Here's the drawing with two shaded views (mm, measured from the low corner). I have some questions. A direction names the side the tool comes from. Give positions to 0.01 mm unless a question says otherwise; leave off trailing zeros. Loops run counter-clockwise (first coordinate to the right, second up) from the corner with the lowest first, then second, coordinate; pieces in that order, holes last. Notation, with made-up numbers: M 56,49.5 L 112,49.5 A10 ccw 112,65.5 Z; hole C 40.25,20.25 d8. An arc over 180 degrees is marked long. Use a Markdown table: item, result. Add a question column.
1) Which directions (+Z, -Z, +X, -X, +Y, -Y) give clear straight access to the entire face, cutting with the end or side of a thin tool? Please do the marked faces 4, 5 and 6.
2) If I drill on line 1 along Z through (x, y) = (37.5, 3.5); line 2 along Z through (x, y) = (47.5, 22.5); line 3 along X through (y, z) = (36.5, 5), over which ranges is the centre line in solid material (lowest first)? Write a range as [from, to].
3) We'd pull the mould along Z, two halves only. Please class the marked faces 1, 2 and 3: +Z half, -Z half, draft (parallel to the pull), parting line (faces both ways), or undercut.
4) Suppose I cut it at A-A on x = 34. List the corners of the cut face in (y, z) for me.
5) Will these pins go through, and if not, where does the flat tip stop? pin 1 Ø9.5 at (x, y) = (16.5, 5.5) entering from -Z; pin 2 Ø0.9 at (y, z) = (37, 5.5) entering from +X; pin 3 Ø2 at (x, z) = (61.5, 19) entering from +Y.
6) Suppose I cut it at D-D on z = 19.5. List the corners of the cut face in (x, y) for me.
7) Suppose I cut it at C-C on y = 24.5. List the corners of the cut face in (x, z) for me.
8) Suppose I cut it at B-B on z = 12. List the corners of the cut face in (x, y) for me.
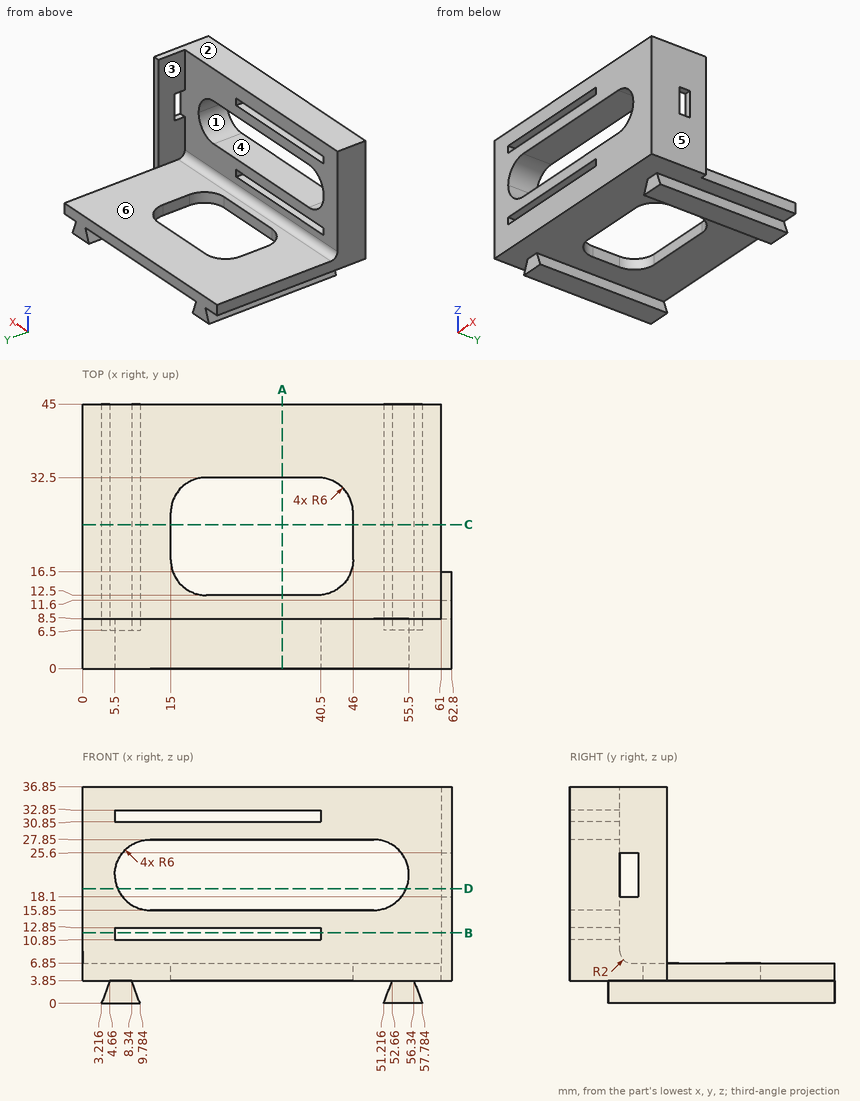
Answer block:
| question | item | result |
|---|---|---|
| 1 | face 4 | +Y, -Y |
| 1 | face 5 | +Z, -Z, +X, +Y, -Y |
| 1 | face 6 | +Z, -X, +Y |
| 2 | line 1 | z = [3.85, 10.85], [12.85, 15.85], [27.85, 30.85], [32.85, 36.85] |
| 2 | line 2 | z = [3.85, 6.85] |
| 2 | line 3 | x = [0, 61] |
| 3 | face 1 | undercut |
| 3 | face 2 | +Z half |
| 3 | face 3 | draft |
| 4 | outline | M 0,3.85 L 12.5,3.85 L 12.5,6.85 L 10.5,6.85 A2 cw 8.5,8.85 L 8.5,10.85 L 0,10.85 Z; M 0,12.85 L 8.5,12.85 L 8.5,15.85 L 0,15.85 Z; M 0,27.85 L 8.5,27.85 L 8.5,30.85 L 0,30.85 Z; M 0,32.85 L 8.5,32.85 L 8.5,36.85 L 0,36.85 Z; M 32.5,3.85 L 45,3.85 L 45,6.85 L 32.5,6.85 Z |
| 5 | pin 1 | stops at z = 3.85 |
| 5 | pin 2 | stops at x = 61 |
| 5 | pin 3 | stops at y = 16.5 |
| 6 | outline | M 0,0 L 5.98,0 L 5.98,8.5 L 0,8.5 Z; M 55.02,0 L 62.8,0 L 62.8,8.5 L 55.02,8.5 Z; M 61,11.6 L 62.8,11.6 L 62.8,16.5 L 61,16.5 Z |
| 7 | outline | M 0,3.85 L 4.66,3.85 L 3.22,0 L 9.78,0 L 8.34,3.85 L 15,3.85 L 15,6.85 L 0,6.85 Z; M 46,3.85 L 52.66,3.85 L 51.22,0 L 57.78,0 L 56.34,3.85 L 61,3.85 L 61,6.85 L 46,6.85 Z |
| 8 | outline | M 0,0 L 5.5,0 L 5.5,8.5 L 0,8.5 Z; M 40.5,0 L 62.8,0 L 62.8,16.5 L 61,16.5 L 61,8.5 L 40.5,8.5 Z |
